Here's how the part is built. I have some questions about the finished solid (model axes, mm). A direction names the side the tool comes from. Give positions to 0.01 mm unless a question says otherwise; leave off trailing zeros. Loops run counter-clockwise (first coordinate to the right, second up) from the corner with the lowest first, then second, coordinate; pieces in that order, holes last. Notation, with made-up numbers: (77, -18.5) - (120, -18.5) arc R20 ccw to (120, -3.5) - close; hole circle Ø8 at (24, 89.5). An arc over 180 degrees is marked (long way). Use a Markdown table: item, result.
from build123d import *

# Parameters (mm, degrees)
SKETCH1_W                = 914.4
SKETCH1_H                = 609.6
SKETCH1_W_2              = 824.59743879
SKETCH1_H_2              = 519.79743879
BOSS_EXTRUDE1_DEPTH      = 101.6
SKETCH2_W                = 914.4
SKETCH2_H                = 609.6
BOSS_EXTRUDE2_DEPTH      = 2.54
BOSS_EXTRUDE3_REACH      = 1116.579
SKETCH4_W                = 914.4
SKETCH4_H                = 609.6
SKETCH4_W_2              = 386.898719395
SKETCH4_H_2              = 519.79743879
BOSS_EXTRUDE4_DEPTH      = 34.925
BOSS_EXTRUDE5_DEPTH      = 0.0254
BOSS_EXTRUDE5_DEPTH_BACK = 6.35
SKETCH5_W                = 386.898719395
SKETCH5_H                = 519.79743879


with BuildPart() as part:
    # Sketch1 → Boss-Extrude1 (new body)
    with BuildSketch(Plane.XY):
        with Locations((457.2, 304.8)):
            Rectangle(SKETCH1_W, SKETCH1_H)
        with Locations((457.2, 304.8)):
            Rectangle(SKETCH1_W_2, SKETCH1_H_2, mode=Mode.SUBTRACT)
    extrude(amount=BOSS_EXTRUDE1_DEPTH)

    # Sketch3 → Boss-Extrude3 (add, up to next)
    with BuildSketch(Plane(origin=(0, 44.901280605, 0), x_dir=(1, 0, 0), z_dir=(0, 1, 0)), mode=Mode.PRIVATE) as boss_extrude3_sk1:
        Polygon((457.2, 0), (482.6, 0), (482.6, -101.6), (431.8, -101.6), (431.8, 0), align=None)
    boss_extrude3_tool1 = extrude(boss_extrude3_sk1.sketch, amount=BOSS_EXTRUDE3_REACH, mode=Mode.PRIVATE) - part.part
    add(boss_extrude3_tool1.solids().sort_by_distance((457.2, 44.901281, 50.8))[0])



with BuildPart() as body_2:
    # Sketch2 → Boss-Extrude2 (new body)
    with BuildSketch(Plane.XY.offset(101.6)):
        Polygon((0, 635), (939.8, 635), (939.8, -25.4), (-25.4, -25.4), (-25.4, 635), align=None)
        with Locations((457.2, 304.8)):
            Rectangle(SKETCH2_W, SKETCH2_H, mode=Mode.SUBTRACT)
    extrude(amount=BOSS_EXTRUDE2_DEPTH)


with BuildPart() as part_1:
    add(part.part)

    add(body_2.part)  # Boss-Extrude4 merges body 2
    # Sketch4 → Boss-Extrude4 (add)
    with BuildSketch(Plane.XY.offset(101.6)):
        with Locations((457.2, 304.8)):
            Rectangle(SKETCH4_W, SKETCH4_H)
        with Locations((238.350640303, 304.8)):
            Rectangle(SKETCH4_W_2, SKETCH4_H_2, mode=Mode.SUBTRACT)
        with Locations((676.049359697, 304.8)):
            Rectangle(SKETCH4_W_2, SKETCH4_H_2, mode=Mode.SUBTRACT)
    extrude(amount=BOSS_EXTRUDE4_DEPTH)

    # Sketch5 → Boss-Extrude5 (add, two sides: drawn at the far end of the back side and taken through both)
    with BuildSketch(Plane(origin=(0, 0, 0), x_dir=(-1, 0, 0), z_dir=(0, 0, -1)).offset(-BOSS_EXTRUDE5_DEPTH_BACK)):
        with Locations((-676.049359697, 304.8)):
            Rectangle(SKETCH5_W, SKETCH5_H)
        with Locations((-238.350640303, 304.8)):
            Rectangle(SKETCH5_W, SKETCH5_H)
    extrude(amount=BOSS_EXTRUDE5_DEPTH + BOSS_EXTRUDE5_DEPTH_BACK)


solid = part_1.part
(1) Suppose I cut it at C-C on x = 775. Write out the boundary of the cut face in (y, z) (3 decimals).
A:
| item | result |
|---|---|
| outline | (-25.4, 101.6) - (0, 101.6) - (0, 0) - (44.901, 0) - (44.901, -0.025) - (564.699, -0.025) - (564.699, 0) - (609.6, 0) - (609.6, 101.6) - (635, 101.6) - (635, 104.14) - (609.6, 104.14) - (609.6, 136.525) - (564.699, 136.525) - (564.699, 6.35) - (44.901, 6.35) - (44.901, 136.525) - (0, 136.525) - (0, 104.14) - (-25.4, 104.14) - close |
(2) Suppose I cut it at A-A on z = 19. Write out the boundary of the cut face in (x, y), plus the area to 3 significant figures.
A:
| item | result |
|---|---|
| outline | (0, 0) - (914.4, 0) - (914.4, 609.6) - (0, 609.6) - close; hole (44.9, 44.9) - (431.8, 44.9) - (431.8, 564.7) - (44.9, 564.7) - close; hole (482.6, 44.9) - (869.5, 44.9) - (869.5, 564.7) - (482.6, 564.7) - close |
| area | 155,000 mm2 |
(3) If I drill on line 1 (X direction, y = 89, z = 100.5); line 2 (X direction, y = 358.5, z = 103); line 3 (Y direction, x = 68.5, z = 81), over which ranges is the centre line in solid material (lowest first)?
A:
| item | result |
|---|---|
| line 1 | 0 to 44.9, 431.8 to 482.6, 869.5 to 914.4 |
| line 2 | -25.4 to 44.9, 431.8 to 482.6, 869.5 to 939.8 |
| line 3 | 0 to 44.9, 564.7 to 609.6 |
(4) On a 3-axis mill with a long thin cutter (end or side, diameter ignored), from which of +Z, -Z, +X, -X, +Y, -Y can I reach the whole of each face in a straight line? I mean faces 4 (the face through (673, 564.699, 71)), 5 (the face through (451, 609.6, 120)), 6 (the face through (451, 0, 50)). Say none if no direction works.
A:
| item | result |
|---|---|
| face 4 | +Z |
| face 5 | +Z, +X, -X, +Y |
| face 6 | -Z, +X, -X, -Y |
(5) We'd pull the mould along X, two halves only. Please class faces 1 (the face through (236, 564.699, 71)), 2 (the face through (451, 609.6, 50)), 3 (the face through (914.4, 301, 120)): pulls with the +X half, pulls with the -X half, needs draft (parallel to the pull), parting line crosses it, or undercut.
A:
| item | result |
|---|---|
| face 1 | undercut |
| face 2 | needs draft |
| face 3 | pulls with the +X half |
(6) Will these pins go through, and if not, where does the flat tip stop? pin 1 (8 mm diameter, centred on y = 494, z = 35, fed in from -X); pin 2 (9.5 mm diameter, centred on y = 419, z = 124, fed in from +X); pin 3 (3 mm diameter, centred on x = 319.5, y = 403, fed in from +Z).
A:
| item | result |
|---|---|
| pin 1 | x = 0 |
| pin 2 | x = 914.4 |
| pin 3 | z = 6.35 |
(7) Suppose I cut it at B-B on y = 33.5. Write out the boundary of the cut face in (x, z) (3 decimals).
A:
| item | result |
|---|---|
| outline | (-25.4, 101.6) - (0, 101.6) - (0, 0) - (914.4, 0) - (914.4, 101.6) - (939.8, 101.6) - (939.8, 104.14) - (914.4, 104.14) - (914.4, 136.525) - (0, 136.525) - (0, 104.14) - (-25.4, 104.14) - close |
(8) Suppose I cut it at D-D on y = 222. Write out the boundary of the cut face in (x, z) (3 decimals).
A:
| item | result |
|---|---|
| outline | (-25.4, 101.6) - (0, 101.6) - (0, 0) - (44.901, 0) - (44.901, -0.025) - (431.8, -0.025) - (431.8, 0) - (482.6, 0) - (482.6, -0.025) - (869.499, -0.025) - (869.499, 0) - (914.4, 0) - (914.4, 101.6) - (939.8, 101.6) - (939.8, 104.14) - (914.4, 104.14) - (914.4, 136.525) - (869.499, 136.525) - (869.499, 6.35) - (482.6, 6.35) - (482.6, 136.525) - (431.8, 136.525) - (431.8, 6.35) - (44.901, 6.35) - (44.901, 136.525) - (0, 136.525) - (0, 104.14) - (-25.4, 104.14) - close |
